Could you check a few things on this model? Use its own coordinates, in mm. A direction names the side the tool comes from. Round coordinates to 2 decimals unless told otherwise and drop trailing zeros. Loops run counter-clockwise (first coordinate to the right, second up) from the corner with the lowest first, then second, coordinate; pieces in that order, holes last. Notation, with made-up numbers: (-30.5, 48) -> (26.5, 48) arc R26 cw to (26.5, 85) -> close; hole circle Ø11 at (61, 0). An arc over 180 degrees is marked (long way). One line per item, written item: value.
from build123d import *

# Parameters (mm, degrees)
F0_W     = 137.495763
F0_H     = 137.29991
F1_DEPTH = 25.4
F2_DEPTH = 3.81
F3_DEPTH = 3.81
F5_D     = 15.24
F5_DEPTH = 12.7
F7_D     = 15.7988
F7_DEPTH = 12.7
F9_D     = 15.7988
F9_DEPTH = 12.7


with BuildPart() as f1:
    # F0 (on Top) → F1 (new body)
    with BuildSketch(Plane.XY):
        with Locations((2.350356, 0.783451)):
            Rectangle(F0_W, F0_H)
        Polygon((-62.872, 59.248533), (-62.872, 65.320283), (-56.996111, 65.320283), (67.964435, 65.320283), (67.964435, -58.269218), (67.964435, -63.165791), (59.93405, -63.165791), (-62.872, -63.165791), align=None, mode=Mode.SUBTRACT)
        Polygon((-56.996111, 65.320283), (-62.872, 65.320283), (-62.872, 59.248533), (59.93405, -63.165791), (67.964435, -63.165791), (67.964435, -58.269218), align=None)
    extrude(amount=F1_DEPTH)

    # F0 (on Top) → F2 (join)
    with BuildSketch(Plane.XY):
        Polygon((67.964435, 65.320283), (-56.996111, 65.320283), (67.964435, -58.269218), align=None)
    extrude(amount=F2_DEPTH)

    # F0 (on Top) → F3 (join)
    with BuildSketch(Plane.XY):
        Polygon((59.93405, -63.165791), (-62.872, 59.248533), (-62.872, -63.165791), align=None)
    extrude(amount=F3_DEPTH)

    # F5
    with Locations(Plane.YZ.offset(71.098238)):
        with Locations((37.975904, 13.292117)):
            Hole(F5_D / 2, depth=F5_DEPTH)

    # F7
    with Locations(Plane(origin=(-66.397525, 0, 0), x_dir=(0, -1, 0), z_dir=(-1, 0, 0))):
        with Locations((37.605681, 13.612472)):
            Hole(F7_D / 2, depth=F7_DEPTH)

    # F9
    with Locations(Plane(origin=(-1.711451, -1.716927, 0), x_dir=(0.708235, -0.705976, 0), z_dir=(-0.705976, -0.708235, 0))):
        with Locations((3.334498, 12.943435)):
            Hole(F9_D / 2, depth=F9_DEPTH)


solid = f1.part
(1) I'm going to push flat-ended pins straight in: pin 1 Ø8 at (x, y) = (38, -14.5) entering from +Z; pin 2 Ø9 at (y, z) = (37.98, 13.29) entering from +X. Where does each tip first touch, or does it pass through?
Recorded:
pin 1: z = 3.81
pin 2: x = -24.8
(2) For faces 1 (the face through (-2.33, -1.1, 21.65)), 2 (the face through (1, 2, 0)), 3 (the face through (-64.61, -30.071, 15.985)), which set-ups out of +Z, -Z, +X, -X, +Y, -Y let a thin tool reach every point of the face, with its end or its side?
Recorded:
face 1: +Z
face 2: -Z, +X, -X, +Y, -Y
face 3: -X
(3) If we section it at D-D, the plane x = -54.5: Please give me the cut outline in (y, z).
Recorded:
outline: (-67.87, 0) -> (69.43, 0) -> (69.43, 25.4) -> (65.32, 25.4) -> (65.32, 3.81) -> (62.85, 3.81) -> (62.85, 25.4) -> (50.9, 25.4) -> (50.9, 3.81) -> (-63.17, 3.81) -> (-63.17, 25.4) -> (-67.87, 25.4) -> close
(4) If we section it at C-C, the plane z = 7.5: Please give me the cut outline in (x, y), then the cut area to 3 significant figures.
Recorded:
outline: (-66.4, -67.87) -> (71.1, -67.87) -> (71.1, 33.02) -> (67.96, 33.02) -> (67.96, -58.27) -> (10.93, -1.86) -> (4.7, -8.11) -> (59.93, -63.17) -> (-62.87, -63.17) -> (-62.87, -42.61) -> (-66.4, -42.61) -> close; (-66.4, -32.6) -> (-62.87, -32.6) -> (-62.87, 59.25) -> (-3.4, -0.03) -> (2.79, 6.19) -> (-57, 65.32) -> (67.96, 65.32) -> (67.96, 42.93) -> (71.1, 42.93) -> (71.1, 69.43) -> (-66.4, 69.43) -> close
area: 3,470 mm²
(5) If we section it at A-A, the plane z = 23.5: Please give me the cut outline in (x, y).
Recorded:
outline: (-66.4, -67.87) -> (71.1, -67.87) -> (71.1, 69.43) -> (-66.4, 69.43) -> close; hole (-62.87, -63.17) -> (59.93, -63.17) -> (-62.87, 59.25) -> close; hole (-57, 65.32) -> (67.96, -58.27) -> (67.96, 65.32) -> close
(6) If we section it at B-B, the plane y = 37: Please give me the cut outline in (x, z), then the cut area to 3 significant figures.
Recorded:
outline: (-66.4, 0) -> (71.1, 0) -> (71.1, 5.73) -> (67.96, 5.73) -> (67.96, 3.81) -> (-28.36, 3.81) -> (-28.36, 25.4) -> (-40.55, 25.4) -> (-40.55, 3.81) -> (-62.87, 3.81) -> (-62.87, 25.4) -> (-66.4, 25.4) -> close; (67.96, 20.85) -> (71.1, 20.85) -> (71.1, 25.4) -> (67.96, 25.4) -> close
area: 883 mm²
(7) Thinking about a two-plate mould opening in Z: for faces 4 (the face through (69.51, 30.94, 10.37)), 5 (the face through (1, 69.433, 13)), 6 (the face through (2, 1, 25.4)), which applies, released by +Z, released by -Z, zero draft, split by the parting line, or undercut?
Recorded:
face 4: undercut
face 5: zero draft
face 6: released by +Z
(8) If I drill on L1, parallel to Y at x = 49, z = 22; L2, parallel to X at y = -12, z = 20.5; L3, parallel to Y at x = 46.5, z = 18.5, over which ranges is the centre line in solid material (lowest first)?
Recorded:
L1: -67.87 to -63.17, -52.27 to -39.51, 65.32 to 69.43
L2: -66.4 to -62.87, 8.6 to 21.18, 67.96 to 71.1
L3: -67.87 to -63.17, -49.77 to -37.04, 65.32 to 69.43
